Part model, mm, in its own coordinate system. A direction names the side the tool comes from. Give positions to 0.01 mm unless a question says otherwise; leave off trailing zeros. Write each loop counter-clockwise with the first axis right and the second up, starting at its lowest first coordinate (ties: lowest second). Pieces come first, ordered by that corner, then holes. Notation, with made-up numbers: M -11.5,29 L -1.5,29 A25 cw -1.5,67 Z; hole C 57,10 d10. An arc over 180 degrees is marked long. Use CSV: the item, a comma, the result in double quotes. Start each with the question number.
1. Band-saw the part on D-D, the plane z = -7. List the corners of the cut face in (x, y).
2. Band-saw the part on A-A, the plane x = 0. List the corners of the cut face in (y, z), then the cut area to 3 significant figures.
3. Band-saw the part on B-B, the plane z = -30.63. List the corners of the cut face in (x, y).
4. Band-saw the part on C-C, the plane x = -30.63. List the corners of the cut face in (y, z).
5. Drill centre lines: line 1 along Z through (x, y) = (30.63, -92.7); line 2 along Y through (x, z) = (17.5, 8); line 3 along Y through (x, z) = (-19, -22). Where is each one in solid material? Low to high. Write a range as from..to.
6. Drop flat-ended pins along their axis: pin 1 Ø2 at (y, z) = (-95.5, -6.5) entering from +X; pin 2 Ø1 at (x, y) = (-20.5, -101.5) entering from -Z; pin 3 Ø10 at (x, z) = (-6, 27) entering from -Y; pin 4 Ø1.6 at (x, z) = (-30.63, 30.63) entering from -Y. Give the stop position or say it passes through.
7. 3-axis set-ups, long thin cutter, end or side, ignore diameter. For faces 1 (the face through (-20, -100, 0)), 2 (the face through (9.1, -98.89, -16.99)), 3 (the face through (-2.248, -97.878, -17.125)), 4 (the face through (-8, -91.81, 16)), 5 (the face through (-8.878, -105.195, 17.105)): which of +Z, -Z, +X, -X, +Y, -Y reach the whole face in a straight line?
8. Mould opens along X. For faces 6 (the face through (12.185, -99.969, 16.219)), 7 (the face through (0, -93, -34.466)), 8 (the face through (16.476, -107.318, 5.188)) say: pulls with the +X half, pulls with the -X half, needs draft (parallel to the pull), parting line crosses it, or undercut.
Autodesk Inventor part; units mm, degrees
ref_plane "Work Plane1" through (-148.5253, -91.81, -70.5943) normal (0, -1, 0) x (1, 0, 0)
ref_plane "Work Plane3" through (-148.5253, -93.81, -70.5943) normal (0, -1, 0) x (1, 0, 0)
ref_plane "Work Plane2" through (-148.5253, -93.81, -70.5943) normal (0, -1, 0) x (1, 0, 0)
ref_plane "Work Plane1" through (-148.5253, -91.81, -70.5943) normal (0, -1, 0) x (1, 0, 0)
sketch "Sketch6" plane through (-148.5253, -91.81, -70.5943) normal (0, -1, 0) x (1, 0, 0)
  line L0 (182.9917, 36.1279) -> (114.0589, 36.1279)
  line L1 (182.9917, 105.0607) -> (182.9917, 36.1279)
  line L2 (114.0589, 36.1279) -> (114.0589, 105.0607)
  line L3 (114.0589, 105.0607) -> (182.9917, 105.0607)
  circle A0 centre (179.1553, 101.2243) radius 1
  circle A1 centre (117.8953, 101.2243) radius 1
  circle A2 centre (117.8953, 39.9643) radius 1
  circle A3 centre (179.1553, 39.9643) radius 1
  point P0 (148.5253, 70.5943)
extrude "Extrusion1" add sketch "Sketch6" along normal blind 2
ref_plane "Work Plane3" through (-148.5253, -93.81, -70.5943) normal (0, -1, 0) x (1, 0, 0)
sketch "Sketch7" plane through (-148.5253, -93.81, -70.5943) normal (0, -1, 0) x (1, 0, 0)
  circle A0 centre (148.5253, 70.5943) radius 17.272
  dimension "d3" = 34.544
extrude "Extrusion2" cut sketch "Sketch7" against normal blind 2
ref_plane "Work Plane2" through (-148.5253, -93.81, -70.5943) normal (0, -1, 0) x (1, 0, 0)
sketch "Sketch8" plane through (-148.5253, -93.81, -70.5943) normal (0, -1, 0) x (1, 0, 0)
  circle A0 centre (148.5253, 70.5943) radius 19.272
  circle A1 centre (148.5253, 70.5943) radius 17.272
  dimension "d6" = 2
extrude "Extrusion3" add sketch "Sketch8" along normal blind 10.3076
sketch "Sketch9" plane through (-148.5253, -93.81, -70.5943) normal (0, -1, 0) x (1, 0, 0)
  arc A0 (160.2004, 63.2971) -> (137.9644, 32.6515) centre (152.0021, 45.8559) ccw
  circle A1 centre (148.5253, 70.5943) radius 19.272
  arc A2 (161.3025, 87.6014) -> (127.2533, 70.5943) centre (148.5253, 70.5943) ccw
  line L0 (129.2533, 70.5943) -> (127.2533, 70.5943)
  line L1 (161.3025, 87.6014) -> (160.1012, 86.0024)
  dimension "d9" = 2
  dimension "d10" = 1.599
ref_plane "Work Plane4" through (79.84, -63.33, -9.91) normal (-1, 0, 0) x (0, 1, 0)
sketch "Sketch10" plane through (79.84, -63.33, -9.91) normal (-1, 0, 0) x (0, 1, 0)
  line L0 (-30.48, -44.3764) -> (-30.48, 24.5564) construction
  line L1 (-40.7876, 9.362) -> (-40.7876, -29.182) construction
  line L2 (-42.7826, 28.0328) -> (-42.7826, -4.4435) construction
  point P0 (63.33, -9.91)
  dimension "d11" = 10.3076
  dimension "d12" = 12.3026
extrude "Extrusion4" add sketch "Sketch9" along normal blind 12.4936 contours A1 L0 A2 L1
sketch "Sketch11" plane through (-148.5253, -106.3036, -70.5943) normal (0, -1, 0) x (1, 0, 0)
  arc A0 (236.18, 74.3245) -> (238.4751, 66.3206) centre (237.3276, 70.3226) ccw construction
  line L0 (236.18, 74.3245) -> (189.5181, 60.9444) construction
  arc A1 (160.2004, 63.2971) -> (189.5181, 60.9444) centre (177.9908, 101.1449) ccw construction
  arc A2 (160.2004, 63.2971) -> (137.9644, 32.6515) centre (152.0021, 45.8559) ccw construction
  line L1 (136.5076, 31.2812) -> (137.9644, 32.6515) construction
  arc A3 (136.5076, 31.2812) -> (169.8778, 34.3252) centre (152.0021, 45.8559) ccw construction
  arc A4 (172.0656, 37.3886) -> (169.8778, 34.3252) centre (203.3405, 12.74) ccw construction
  line L2 (170.4948, 38.6266) -> (172.0656, 37.3886) construction
  arc A5 (191.8132, 52.9405) -> (170.4948, 38.6266) centre (203.3405, 12.74) ccw construction
  line L3 (191.8132, 52.9405) -> (238.4751, 66.3206) construction
  line L4 (129.2533, 70.5943) -> (127.2533, 70.5943) construction
  line L5 (129.2533, 70.5943) -> (165.4777, 70.5943) construction
  circle A6 centre (148.5253, 70.5943) radius 17.272 construction
  line L6 (148.5253, 87.8663) -> (148.5253, 53.3223) construction
  circle A7 centre (148.5253, 70.5943) radius 17.272 construction
  circle A8 centre (148.5253, 70.5943) radius 19.272 construction
  circle A9 centre (148.5253, 70.5943) radius 21.272
  dimension "d15" = 42.544
extrude "Extrusion5" add sketch "Sketch11" along normal blind 2
sketch "Sketch12" plane through (0, -108.3036, 0) normal (0, -1, 0) x (1, 0, 0)
  circle A0 centre (0, 0) radius 17.2734
extrude "Extrusion6" cut sketch "Sketch12" against normal blind 2
properties part number "TrapAdapter" material "ABS Plastic"
Output:
1,outline,"M -34.47,-93.81 L -17.96,-93.81 L -17.96,-104.12 L -15.79,-104.12 L -15.79,-91.81 L -34.47,-91.81 Z; M -20.09,-108.3 L -15.79,-108.3 L -15.79,-106.3 L -20.09,-106.3 Z; M 15.79,-108.3 L 20.09,-108.3 L 20.09,-106.3 L 15.79,-106.3 Z; M 15.79,-104.12 L 17.96,-104.12 L 17.96,-93.81 L 34.47,-93.81 L 34.47,-91.81 L 15.79,-91.81 Z"
2,outline,"M -108.3,-21.27 L -106.3,-21.27 L -106.3,-17.27 L -108.3,-17.27 Z; M -108.3,17.27 L -106.3,17.27 L -106.3,19.27 L -104.12,19.27 L -104.12,17.27 L -91.81,17.27 L -91.81,34.47 L -93.81,34.47 L -93.81,21.27 L -108.3,21.27 Z; M -104.12,-19.27 L -93.81,-19.27 L -93.81,-34.47 L -91.81,-34.47 L -91.81,-17.27 L -104.12,-17.27 Z"
2,area,"151 mm²"
3,outline,"M -34.47,-93.81 L -31.63,-93.81 L -31.63,-91.81 L -34.47,-91.81 Z; M -29.63,-93.81 L 29.63,-93.81 L 29.63,-91.81 L -29.63,-91.81 Z; M 31.63,-93.81 L 34.47,-93.81 L 34.47,-91.81 L 31.63,-91.81 Z"
4,outline,"M -93.81,-34.47 L -91.81,-34.47 L -91.81,-31.63 L -93.81,-31.63 Z; M -93.81,-29.63 L -91.81,-29.63 L -91.81,29.63 L -93.81,29.63 Z; M -93.81,31.63 L -91.81,31.63 L -91.81,34.47 L -93.81,34.47 Z"
5,line 1,"z = -34.47..-31.63, -29.63..29.63, 31.63..34.47"
5,line 2,"y = -108.3..-106.3, -104.12..-91.81"
5,line 3,"y = -93.81..-91.81"
6,pin 1,"stops at x = 18.47"
6,pin 2,"stops at z = 0"
6,pin 3,"stops at y = -93.81"
6,pin 4,"passes through"
7,face 1,"-Z, -X"
7,face 2,"none"
7,face 3,"+Y, -Y"
7,face 4,"+Z, -Z, +X, -X, +Y"
7,face 5,"-Z"
8,face 6,"pulls with the +X half"
8,face 7,"needs draft"
8,face 8,"undercut"
